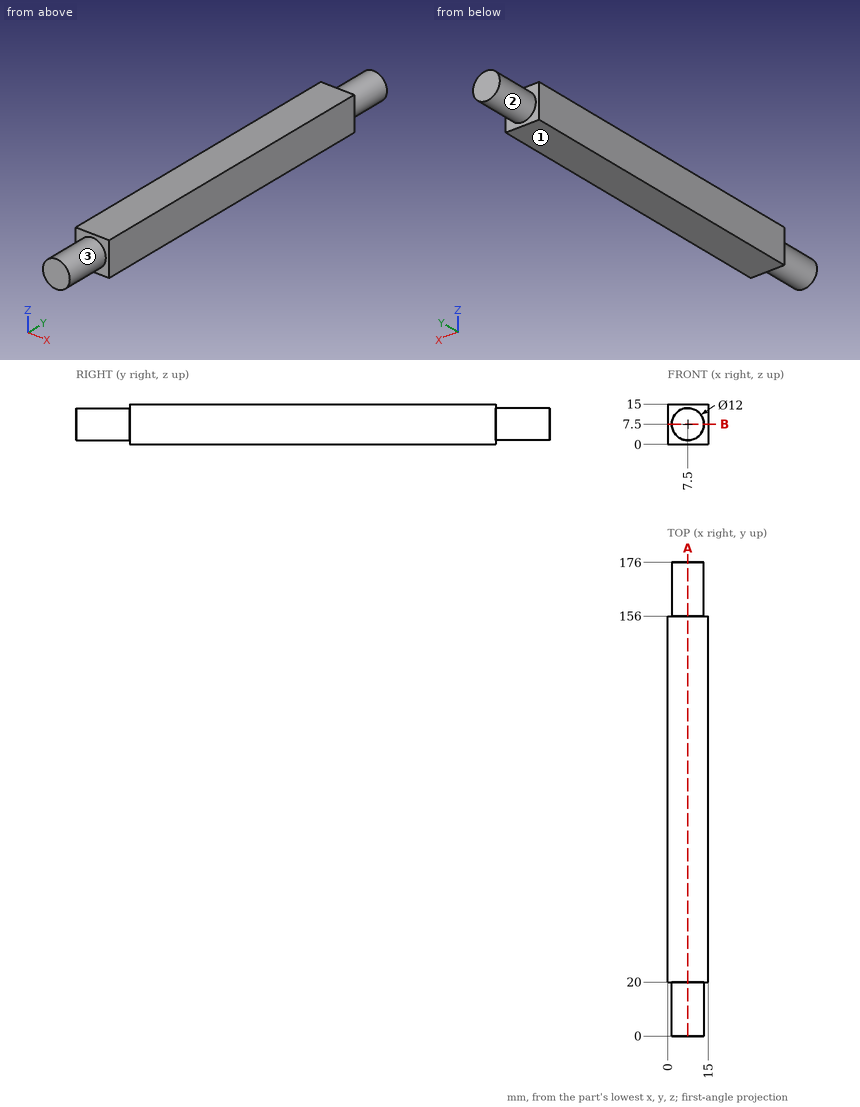
For this review, use the dimensioned drawing (mm, ordinates from the lowest corner) and the shaded views. A direction names the side the tool comes from. Coordinates: 2 decimals unless noted, no trailing zeros. Order: outer loops, then holes, each group sorted by start corner. A loop starts at its lowest first (then second) coordinate and runs counter-clockwise, first axis right, second up. Notation, with made-up numbers: (52.5, 43.5) - (73.5, 43.5) arc R25 cw to (73.5, 70.5) - close; hole circle Ø1 at (4, 50). An arc over 180 degrees is marked (long way). Answer as a JSON object with one key per item and string values. Group by question number.
1. We need section B-B on z = 7.5. State the section outline as (x, y) points, then the cut area to 3 significant figures.
2. For probe 1 along Z at (x, y) = (7, 15); probe 2 along Y at (x, z) = (12.5, 12); probe 3 along X at (y, z) = (13.5, 3), list the stretches that pass through material, from the lowest coordinate up.
3. For the marked faces 1, 2 and 3, list the 3-axis set-ups (+Z, -Z, +X, -X, +Y, -Y) from which the entire face can be reached by the end or side of a thin tool; tool diameter is ignored.
4. We need section A-A on x = 7.5. State the section outline as (y, z) points.
Final values:
{
 "1": {"outline": "(0, 20) - (1.5, 20) - (1.5, 0) - (13.5, 0) - (13.5, 20) - (15, 20) - (15, 156) - (13.5, 156) - (13.5, 176) - (1.5, 176) - (1.5, 156) - (0, 156) - close", "area": "2,520 mm²"},
 "2": {"probe 1": "1.52 to 13.48", "probe 2": "20 to 156", "probe 3": "3.53 to 11.47"},
 "3": {"face 1": "-Z, +X, -X, +Y, -Y", "face 2": "+Y", "face 3": "-Y"},
 "4": {"outline": "(0, 1.5) - (20, 1.5) - (20, 0) - (156, 0) - (156, 1.5) - (176, 1.5) - (176, 13.5) - (156, 13.5) - (156, 15) - (20, 15) - (20, 13.5) - (0, 13.5) - close"}
}
